Check sheet for the modelled part. Datum: model origin and axes. Units: mm. Face numbers are marked on the shaded views. A direction names the side the tool comes from. Round coordinates to 2 decimals unless told otherwise and drop trailing zeros. Order: outer loops, then holes, each group sorted by start corner. A loop starts at its lowest first (then second) coordinate and runs counter-clockwise, first axis right, second up. Notation, with made-up numbers: (-23.5, -9.75) -> (-16.5, -9.75) arc R17 cw to (-16.5, -1.75) -> close; hole circle Ø8 at (5.25, -13). An arc over 180 degrees is marked (long way). Answer in a Markdown table with one row per item.
```python
from build123d import *

# Parameters (mm, degrees)
BOSS_EXTRUDE1_DEPTH = 45.5
SKETCH3_R           = 3.5
CUT_EXTRUDE1_DEPTH  = 46.5
SKETCH5_R           = 50.5
SKETCH5_R_2         = 30
CUT_EXTRUDE2_DEPTH  = 38
SKETCH6_R           = 30
CUT_EXTRUDE3_DEPTH  = 20


with BuildPart() as part:
    # Sketch1 → Boss-Extrude1 (new body)
    with BuildSketch(Plane.XY):
        with BuildLine():
            Line((0, 5), (0, 115))
            ThreePointArc((0, 115), (1.464466094, 118.535533906), (5, 120))
            Line((5, 120), (135, 120))
            ThreePointArc((135, 120), (138.535533906, 118.535533906), (140, 115))
            Line((140, 115), (140, 5))
            ThreePointArc((140, 5), (138.535533906, 1.464466094), (135, 0))
            Line((135, 0), (5, 0))
            ThreePointArc((5, 0), (1.464466094, 1.464466094), (0, 5))
        make_face()
    extrude(amount=BOSS_EXTRUDE1_DEPTH)

    # Sketch3 → Cut-Extrude1 (cut, through all)
    with BuildSketch(Plane.XY.offset(45.5)):
        with Locations((10, 110)):
            Circle(SKETCH3_R)
        with Locations((130, 110)):
            Circle(SKETCH3_R)
        with Locations((10, 10)):
            Circle(SKETCH3_R)
    extrude(amount=-CUT_EXTRUDE1_DEPTH, mode=Mode.SUBTRACT)

    # Sketch5 → Cut-Extrude2 (cut)
    with BuildSketch(Plane.XY.offset(45.5)):
        with Locations((60, 60)):
            Circle(SKETCH5_R)
        with Locations((60, 60)):
            Circle(SKETCH5_R_2, mode=Mode.SUBTRACT)
    extrude(amount=-CUT_EXTRUDE2_DEPTH, mode=Mode.SUBTRACT)

    # Sketch6 → Cut-Extrude3 (cut)
    with BuildSketch(Plane.XY.offset(45.5)):
        with Locations((60, 60)):
            Circle(SKETCH6_R)
    extrude(amount=-CUT_EXTRUDE3_DEPTH, mode=Mode.SUBTRACT)


solid = part.part
```
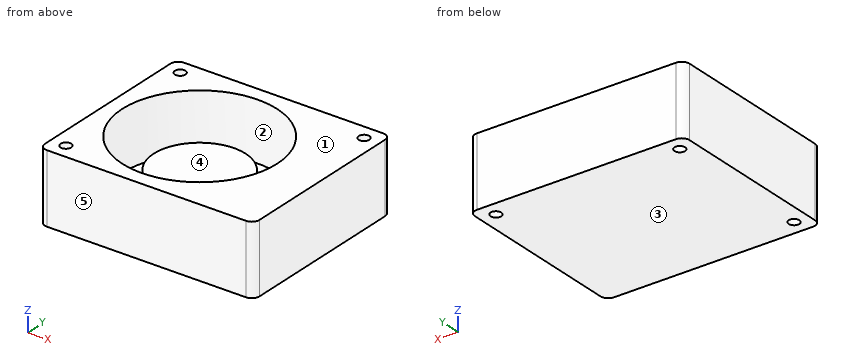
(1) Section check A-A on x = 130. Record the boundary of the cut face in (y, z).
Solutions:
| item | result |
|---|---|
| outline | (0, 0) -> (106.5, 0) -> (106.5, 45.5) -> (0, 45.5) -> close; (113.5, 0) -> (120, 0) -> (120, 45.5) -> (113.5, 45.5) -> close |
(2) Section check D-D on x = 60. Record the boundary of the cut face in (y, z), plus the area to 3 significant figures.
Solutions:
| item | result |
|---|---|
| outline | (0, 0) -> (120, 0) -> (120, 45.5) -> (110.5, 45.5) -> (110.5, 7.5) -> (90, 7.5) -> (90, 25.5) -> (30, 25.5) -> (30, 7.5) -> (9.5, 7.5) -> (9.5, 45.5) -> (0, 45.5) -> close |
| area | 2,700 mm^2 |
(3) Scan lines: probe 1 along Y at (x, z) = (130, 30); probe 2 along Y at (x, z) = (67, 15); probe 3 along Z at (x, y) = (46, 22.5). Record each from-to range of solid material in increasing order. Write a range as from..to.
Solutions:
| item | result |
|---|---|
| probe 1 | 0..106.5, 113.5..120 |
| probe 2 | 0..9.99, 30.83..89.17, 110.01..120 |
| probe 3 | 0..7.5 |
(4) Draft check along Y on the marked faces 3, 4 and 5. Enter one of: pulls with the +Y half, pulls with the -Y half, needs draft (parallel to the pull), parting line crosses it, or undercut.
Solutions:
| item | result |
|---|---|
| face 3 | needs draft |
| face 4 | undercut |
| face 5 | pulls with the -Y half |
(5) Depth check by flat-ended pin: pin 1 Ø1.5 at (x, y) = (61, 71) entering from +Z. Enter the tip coordinate at first touch or a pass-through.
Solutions:
| item | result |
|---|---|
| pin 1 | z = 25.5 |
(6) Section check B-B on z = 34.5. Record the boundary of the cut face in (x, y).
Solutions:
| item | result |
|---|---|
| outline | (0, 5) arc R5 ccw to (5, 0) -> (135, 0) arc R5 ccw to (140, 5) -> (140, 115) arc R5 ccw to (135, 120) -> (5, 120) arc R5 ccw to (0, 115) -> close; hole circle Ø7 at (10, 10); hole circle Ø7 at (10, 110); hole circle Ø101 at (60, 60); hole circle Ø7 at (130, 110) |
(7) Section check C-C on y = 60. Record the boundary of the cut face in (x, z), plus the area to 3 significant figures.
Solutions:
| item | result |
|---|---|
| outline | (0, 0) -> (140, 0) -> (140, 45.5) -> (110.5, 45.5) -> (110.5, 7.5) -> (90, 7.5) -> (90, 25.5) -> (30, 25.5) -> (30, 7.5) -> (9.5, 7.5) -> (9.5, 45.5) -> (0, 45.5) -> close |
| area | 3,610 mm^2 |
(8) Tool access check on the marked faces 1 and 2. Record the directions out of +Z, -Z, +X, -X, +Y, -Y that give a thin tool (end or side, any length) a straight path to the whole face; none if there is none.
Solutions:
| item | result |
|---|---|
| face 1 | +Z, +X, -X, +Y, -Y |
| face 2 | +Z |
